from build123d import *

# Parameters (mm, degrees)
F0_W     = 13
F0_H     = 13
F1_DEPTH = 110
F3_W     = 13
F3_H     = 2.4
F4_DEPTH = 80
F5_T     = -1.6


with BuildPart() as f1:
    # F0 (on Right) → F1 (new body)
    with BuildSketch(Plane.YZ):
        Rectangle(F0_W, F0_H)
    extrude(amount=F1_DEPTH)

    # F3 (on offset) → F4 (cut)
    with BuildSketch(Plane.YZ.offset(110)):
        Rectangle(F3_W, F3_H)
    extrude(amount=-F4_DEPTH, mode=Mode.SUBTRACT)

    # F5 (hollow: no face is removed)
    offset(amount=F5_T, kind=Kind.INTERSECTION, mode=Mode.SUBTRACT)


solid = f1.part
The listing builds one solid part. Answer for the finished solid, in the listing's coordinates (mm). A direction names the side the tool comes from. Give positions to 0.01 mm unless a question says otherwise; leave off trailing zeros. Write each loop counter-clockwise with the first axis right and the second up, starting at its lowest first coordinate (ties: lowest second). Pieces come first, ordered by that corner, then holes.
Item 1: Section A-A, the plane y = 2.25 is taken. Write down the section's boundary in (x, z), plus the area to 3 significant figures.
Item 2: Which of the six approach directions +Z, -Z, +X, -X, +Y, -Y give full straight-line access (tool end or side, diameter ignored) to faces 1 (the flat face through (28.4, 0, 0)), 2 (the flat face through (71, 0, 1.2)), 3 (the flat face through (54, -6.5, -2))?
Item 3: Section D-D, the plane x = 12 is taken. Write down the section's boundary in (y, z).
Item 4: Section B-B, the plane x = 46 is taken. Write down the section's boundary in (y, z).
Item 5: Find the intervals of material crossed by line 1 along Z through (x, y) = (54.5, 0); line 2 along X through (y, z) = (-2.5, 4.75); line 3 along X through (y, z) = (-3, 1), in increasing order.
Item 6: Section C-C, the plane z = 0 is taken. Write down the section's boundary in (x, y), plus the area to 3 significant figures.
Item 7: Flat-ended cylindrical pins translate along their axes: P1, Ø4.5, axis at y = -1, z = 1, coming from the -X side; P2, Ø1.2, axis at y = 0, z = 0.5, coming from the +X side. Find the tip coordinate at first contact, or state that the pin passes through.
Item 8: Determine the mould class of faces 4 (the flat face through (108.4, 0, -4)), 5 (the flat face through (0, 0, 0)), 6 (the flat face through (30, 0, 0)) for opening direction X: released by +X, released by -X, zero draft, split by the parting line, or undercut.
Completed:
1. outline: (0, -6.5) - (110, -6.5) - (110, -1.2) - (30, -1.2) - (30, 1.2) - (110, 1.2) - (110, 6.5) - (0, 6.5) - close; hole (1.6, -4.9) - (108.4, -4.9) - (108.4, -2.8) - (28.4, -2.8) - (28.4, 2.8) - (108.4, 2.8) - (108.4, 4.9) - (1.6, 4.9) - close
1. area: 639 mm2
2. face 1: none
2. face 2: +X, +Y, -Y
2. face 3: +Z, -Z, +X, -X, -Y
3. outline: (-6.5, -6.5) - (6.5, -6.5) - (6.5, 6.5) - (-6.5, 6.5) - close; hole (-4.9, -4.9) - (4.9, -4.9) - (4.9, 4.9) - (-4.9, 4.9) - close
4. outline: (-6.5, -6.5) - (6.5, -6.5) - (6.5, -1.2) - (-6.5, -1.2) - close; (-6.5, 1.2) - (6.5, 1.2) - (6.5, 6.5) - (-6.5, 6.5) - close; hole (-4.9, -4.9) - (4.9, -4.9) - (4.9, -2.8) - (-4.9, -2.8) - close; hole (-4.9, 2.8) - (4.9, 2.8) - (4.9, 4.9) - (-4.9, 4.9) - close
5. line 1: z = -6.5 to -4.9, -2.8 to -1.2, 1.2 to 2.8, 4.9 to 6.5
5. line 2: x = 0 to 1.6, 108.4 to 110
5. line 3: x = 0 to 1.6, 28.4 to 30
6. outline: (0, -6.5) - (30, -6.5) - (30, 6.5) - (0, 6.5) - close; hole (1.6, -4.9) - (28.4, -4.9) - (28.4, 4.9) - (1.6, 4.9) - close
6. area: 127 mm2
7. P1: stops at x = 0
7. P2: stops at x = 30
8. face 4: undercut
8. face 5: released by -X
8. face 6: released by +X
